Verification items for this drawing (mm, ordinates from the low corner). A direction names the side the tool comes from. Round coordinates to 2 decimals unless told otherwise and drop trailing zeros. Loops run counter-clockwise (first coordinate to the right, second up) from the corner with the lowest first, then second, coordinate; pieces in that order, holes last. Notation, with made-up numbers: (-30.75, -5.75) -> (10.25, -5.75) arc R25 ccw to (10.25, 32.25) -> close; hole circle Ø4 at (-24.75, 2.25). An arc over 180 degrees is marked (long way). Use a Markdown table: item, result. Add a question column.
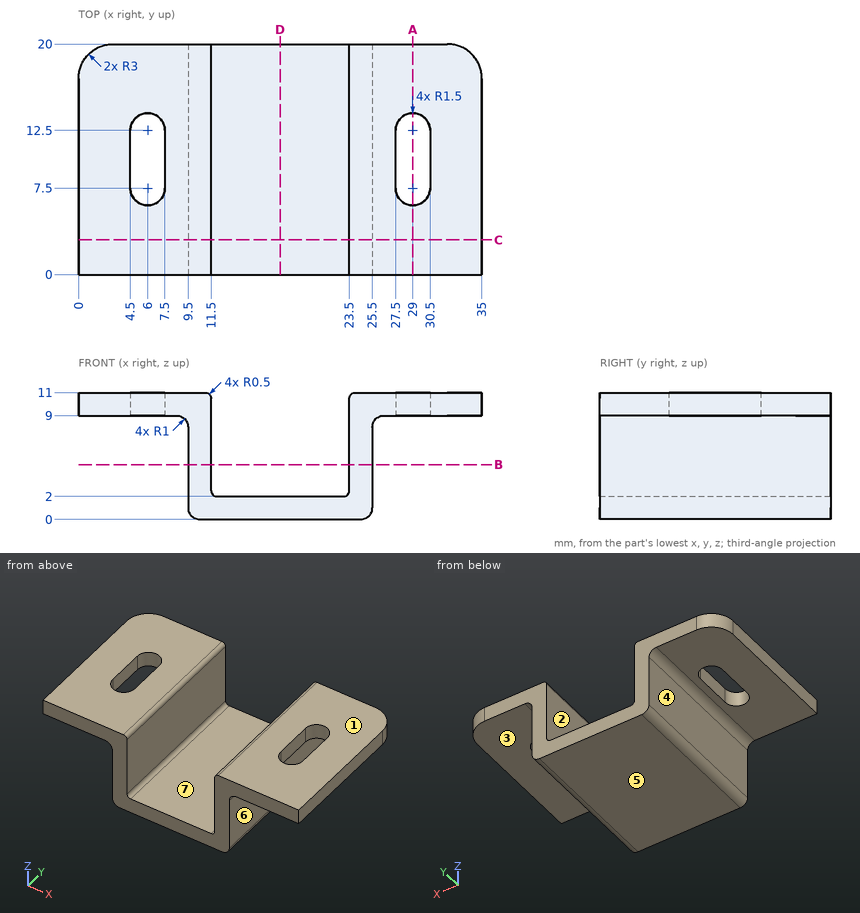
1) Sectioned sample at D-D on x = 17.5. Enter the section's corners in (y, z).
2) Sectioned sample at C-C on y = 3. Enter the section's corners in (x, z), then the cut area to 3 significant figures.
3) Go/stop test with flat-tipped pins: pin 1 (4 mm diameter, centred on x = 3, y = 10, fed in from -Z); pin 2 (4 mm diameter, centred on y = 9.5, z = 6.5, fed in from -X); pin 3 (4 mm diameter, centred on y = 9, z = 5.5, fed in from +X). Record where each tip stops, or that it passes through.
4) Release check for a two-part mould opening along X. For the marked faces 5, 6 and 7 record: released by +X, released by -X, zero draft, split by the parting line, or undercut.
5) Access from +Z, -Z, +X, -X, +Y, -Y to the whole of each face (thin tool, end or side, straight path). Record for the marked faces 1, 2, 3 and 4.
6) Sectioned sample at A-A on x = 29. Enter the section's corners in (y, z), then the cut area to 3 significant figures.
7) Sectioned sample at B-B on z = 4.75. Enter the section's corners in (x, y).
8) Thickness scan on line 1 (X direction, y = 11.5, z = 10.25); line 2 (X direction, y = 13.75, z = 3); line 3 (Z direction, x = 12.5, y = 16). Record the ranges inside material, lowest first.
Geometry results:
| question | item | result |
|---|---|---|
| 1 | outline | (0, 0) -> (20, 0) -> (20, 2) -> (0, 2) -> close |
| 2 | outline | (0, 9) -> (8.5, 9) arc R1 cw to (9.5, 8) -> (9.5, 1) arc R1 ccw to (10.5, 0) -> (24.5, 0) arc R1 ccw to (25.5, 1) -> (25.5, 8) arc R1 cw to (26.5, 9) -> (35, 9) -> (35, 11) -> (24, 11) arc R0.5 ccw to (23.5, 10.5) -> (23.5, 2.5) arc R0.5 cw to (23, 2) -> (12, 2) arc R0.5 cw to (11.5, 2.5) -> (11.5, 10.5) arc R0.5 ccw to (11, 11) -> (0, 11) -> close |
| 2 | area | 106 mm^2 |
| 3 | pin 1 | z = 9 |
| 3 | pin 2 | x = 9.37 |
| 3 | pin 3 | x = 25.5 |
| 4 | face 5 | zero draft |
| 4 | face 6 | released by +X |
| 4 | face 7 | undercut |
| 5 | face 1 | +Z, +X, -X, +Y, -Y |
| 5 | face 2 | +Z, +Y, -Y |
| 5 | face 3 | -Z, +X, +Y, -Y |
| 5 | face 4 | -Z, -X, +Y, -Y |
| 6 | outline | (0, 9) -> (6, 9) -> (6, 11) -> (0, 11) -> close; (14, 9) -> (20, 9) -> (20, 11) -> (14, 11) -> close |
| 6 | area | 24.0 mm^2 |
| 7 | outline | (9.5, 0) -> (11.5, 0) -> (11.5, 20) -> (9.5, 20) -> close; (23.5, 0) -> (25.5, 0) -> (25.5, 20) -> (23.5, 20) -> close |
| 8 | line 1 | 0 to 4.5, 7.5 to 11.5, 23.5 to 27.5, 30.5 to 35 |
| 8 | line 2 | 9.5 to 11.5, 23.5 to 25.5 |
| 8 | line 3 | 0 to 2 |
